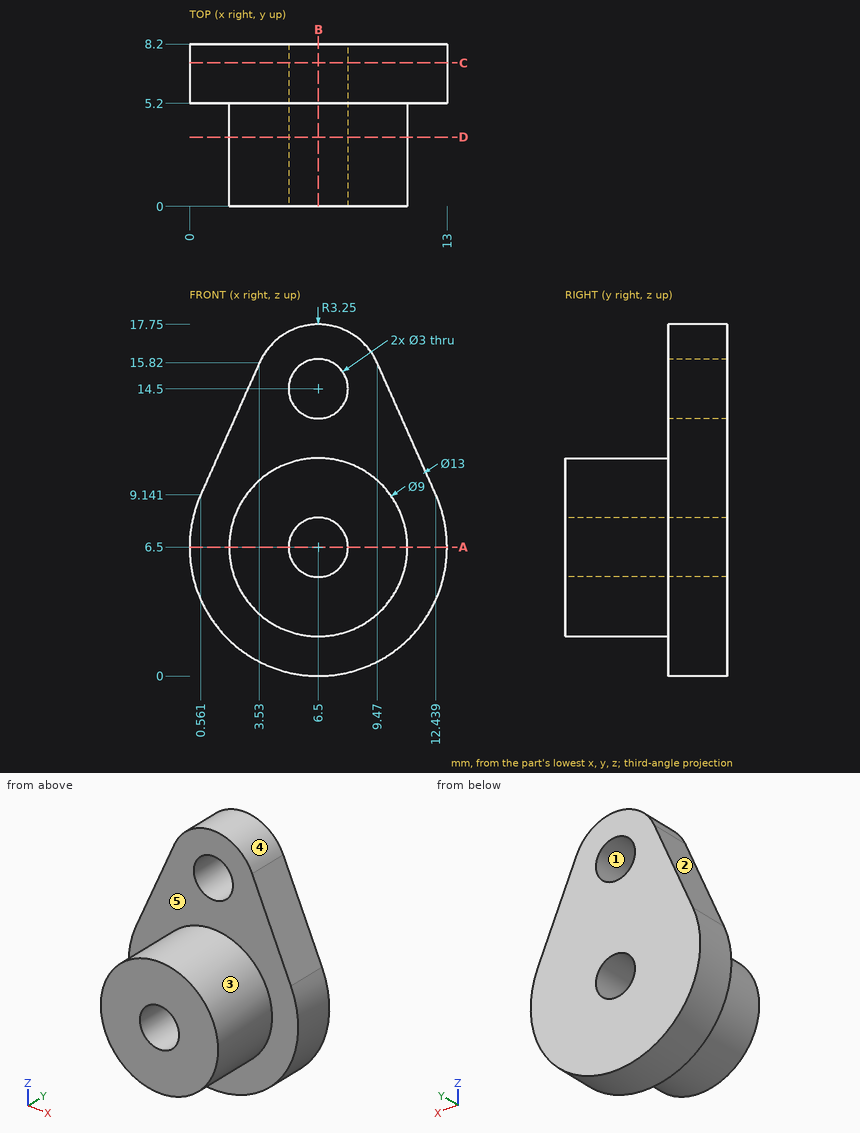
Job drawing, mm, ordinate dimensions from the low corner. One solid piece. A direction names the side the tool comes from. Coordinates: 2 decimals unless noted, no trailing zeros. Order: outer loops, then holes, each group sorted by start corner. A loop starts at its lowest first (then second) coordinate and runs counter-clockwise, first axis right, second up. Notation, with made-up numbers: (63.5, 48.25) -> (83.5, 48.25) arc R11 cw to (83.5, 62.25) -> close; hole circle Ø5 at (74, 38). An arc over 180 degrees is marked (long way). Answer in a Markdown table with one row per item. Add a question column.
Q1. Band-saw the part on C-C, the plane y = 7.25. List the corners of the cut face in (x, z).
Q2. Band-saw the part on D-D, the plane y = 3.5. List the corners of the cut face in (x, z).
Q3. Band-saw the part on A-A, the plane z = 6.5. List the corners of the cut face in (x, y), then the cut area to 3 significant figures.
Q4. Band-saw the part on B-B, the plane x = 6.5. List the corners of the cut face in (y, z).
Q5. Mould opens along Z. For the marked faces 1, 2 and 3 say: +Z half, -Z half, draft (parallel to the pull), parting line (faces both ways), or undercut.
Q6. Which spindle directions (+Z, -Z, +X, -X, +Y, -Y) get a long thin tool onto all of the face, cutting with end or side? Do the marked faces 4 and 5. Say none if no direction does.
Q7. Wall check: line 1 along Z through (x, y) = (6.5, 7.1); line 2 along Z through (x, y) = (7, 6) (1 decimal); line 3 along Y through (x, z) = (7.5, 12.25). Give the ranges that are in metal, low to high. Write a range as [from, to].
Q8. Drop flat-ended pins along their axis: pin 1 (2 mm diameter, centred on y = 2.5, z = 11.5, fed in from -X); pin 2 (2 mm diameter, centred on x = 2, y = 1.5, fed in from -Z); pin 3 (2 mm diameter, centred on y = 3.5, z = 6, fed in from -X). Give the stop position or say it passes through.
Answers follow:
| question | item | result |
|---|---|---|
| 1 | outline | (0.56, 9.14) arc R6.5 ccw (long way) to (12.44, 9.14) -> (9.47, 15.82) arc R3.25 ccw to (3.53, 15.82) -> close; hole circle Ø3 at (6.5, 6.5); hole circle Ø3 at (6.5, 14.5) |
| 2 | outline | circle Ø9 at (6.5, 6.5); hole circle Ø3 at (6.5, 6.5) |
| 3 | outline | (0, 5.2) -> (2, 5.2) -> (2, 0) -> (5, 0) -> (5, 8.2) -> (0, 8.2) -> close; (8, 0) -> (11, 0) -> (11, 5.2) -> (13, 5.2) -> (13, 8.2) -> (8, 8.2) -> close |
| 3 | area | 61.2 mm^2 |
| 4 | outline | (0, 2) -> (5.2, 2) -> (5.2, 0) -> (8.2, 0) -> (8.2, 5) -> (0, 5) -> close; (0, 8) -> (8.2, 8) -> (8.2, 13) -> (5.2, 13) -> (5.2, 11) -> (0, 11) -> close; (5.2, 16) -> (8.2, 16) -> (8.2, 17.75) -> (5.2, 17.75) -> close |
| 5 | face 1 | undercut |
| 5 | face 2 | +Z half |
| 5 | face 3 | parting line |
| 6 | face 4 | +Z, +Y, -Y |
| 6 | face 5 | -Y |
| 7 | line 1 | [0, 5], [8, 13], [16, 17.75] |
| 7 | line 2 | [0, 5.1], [7.9, 13.1], [15.9, 17.7] |
| 7 | line 3 | [5.2, 8.2] |
| 8 | pin 1 | x = 4.44 |
| 8 | pin 2 | z = 3.67 |
| 8 | pin 3 | x = 2 |
